Here's how the part is built. I have some questions about the finished solid (model axes, mm). Give positions to 0.01 mm unless a question says otherwise; leave off trailing zeros. Write each loop counter-clockwise with the first axis right and the second up, starting at its lowest first coordinate (ties: lowest second). Pieces come first, ordered by that corner, then holes. Notation, with made-up numbers: (-27.5, 70.5) -> (6.5, 70.5) arc R17 cw to (6.5, 101.5) -> close; hole circle Ø3 at (-23.5, 66.25). An arc over 180 degrees is marked (long way). Use one line per item in the form item = value.
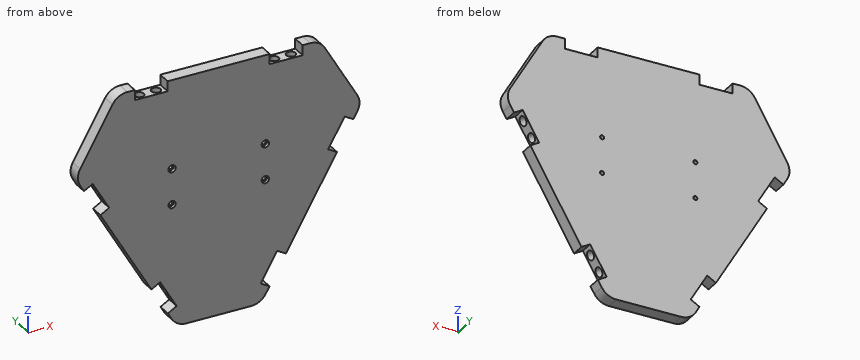
```python
from build123d import *

# Parameters (mm, degrees)
BOSS_EXTRUDE1_DEPTH            = 4
CHAMFER1_SIZE                  = 50
SKETCH4_W                      = 19.5
SKETCH4_H                      = 8
SKETCH4_R                      = 2
CUT_EXTRUDE1_DEPTH             = 6
SKETCH4_2_R                    = 2
CUT_EXTRUDE2_DEPTH             = 16
SKETCH9_R                      = 2.75
CUT_EXTRUDE3_DEPTH             = 7
CRVPATTERN1_START              = -63.508529611
CRVPATTERN1_OUTLINE_W          = 19.5
CRVPATTERN1_OUTLINE_H          = 8
CRVPATTERN1_DEPTH              = 6
CRVPATTERN1_START_2            = -57.508529611
CRVPATTERN1_2_OUTLINE_R        = 2.75
CRVPATTERN1_2_DEPTH            = 7
CRVPATTERN1_START_3            = -50.508529611
CRVPATTERN1_3_OUTLINE_R        = 2
CRVPATTERN1_3_DEPTH            = 3
CRVPATTERN1_START_4            = 57.508529611
CRVPATTERN1_4_OUTLINE_W        = 19.5
CRVPATTERN1_4_OUTLINE_H        = 8
CRVPATTERN1_4_DEPTH            = 6
CRVPATTERN1_START_5            = 50.508529611
CRVPATTERN1_5_OUTLINE_R        = 2.75
CRVPATTERN1_5_DEPTH            = 7
CRVPATTERN1_START_6            = 47.508529611
CRVPATTERN1_6_OUTLINE_R        = 2
CRVPATTERN1_6_DEPTH            = 3
FILLET1_R                      = 10
CBORE_FOR_M2_SHCS1_D           = 2.4
CBORE_FOR_M2_SHCS1_CBORE_D     = 4.4
CBORE_FOR_M2_SHCS1_CBORE_DEPTH = 2


# Read off the part's stored shape, not the designer's step: CrvPattern1
with BuildPart() as part:
    # Sketch1 → Boss-Extrude1 (new, symmetric)
    with BuildSketch(Plane(origin=(0, 0, 0), x_dir=(1, 0, 0), z_dir=(0, 1, 0))):
        Polygon((110, -63.508529611), (0, 127.017059222), (-110, -63.508529611), align=None)
    extrude(amount=BOSS_EXTRUDE1_DEPTH, both=True)

    # Chamfer1
    chamfer1_edges = [part.edges().sort_by_distance(p)[0] for p in [
        (-110, 0, 63.508529611),
        (0, 0, -127.017059222),
        (110, 0, 63.508529611),
    ]]
    chamfer(chamfer1_edges, length=CHAMFER1_SIZE)

    # Sketch4 → Cut-Extrude1 (cut)
    with BuildSketch(Plane(origin=(4.375288244, 0, 63.508529611), x_dir=(-1, 0, 0), z_dir=(0, 0, -1))):
        with Locations((44.375288244, 0)):
            Rectangle(SKETCH4_W, SKETCH4_H)
        with Locations((39.375288244, 0)):
            Circle(SKETCH4_R, mode=Mode.SUBTRACT)
        with Locations((49.375288244, 0)):
            Circle(SKETCH4_R, mode=Mode.SUBTRACT)
    cut_extrude1 = extrude(amount=CUT_EXTRUDE1_DEPTH, mode=Mode.SUBTRACT)

    # Sketch4<2> → Cut-Extrude2 (cut)
    with BuildSketch(Plane(origin=(4.375288244, 0, 63.508529611), x_dir=(-1, 0, 0), z_dir=(0, 0, -1))):
        with Locations((49.375288244, 0)):
            Circle(SKETCH4_2_R)
        with Locations((39.375288244, 0)):
            Circle(SKETCH4_2_R)
    cut_extrude2 = extrude(amount=CUT_EXTRUDE2_DEPTH, mode=Mode.SUBTRACT)

    # Sketch9 → Cut-Extrude3 (cut)
    with BuildSketch(Plane.XY.offset(57.508529611)):
        with Locations((-45, 0)):
            Circle(SKETCH9_R)
        with Locations((-35, 0)):
            Circle(SKETCH9_R)
    cut_extrude3 = extrude(amount=-CUT_EXTRUDE3_DEPTH, mode=Mode.SUBTRACT)

    # Mirror1: Cut-Extrude1, Cut-Extrude2, Cut-Extrude3 across plane
    add(cut_extrude1.mirror(Plane(origin=(0, 0, 0), x_dir=(0, 0, 1), z_dir=(1, 0, 0))), mode=Mode.SUBTRACT)
    add(cut_extrude2.mirror(Plane(origin=(0, 0, 0), x_dir=(0, 0, 1), z_dir=(1, 0, 0))), mode=Mode.SUBTRACT)
    add(cut_extrude3.mirror(Plane(origin=(0, 0, 0), x_dir=(0, 0, 1), z_dir=(1, 0, 0))), mode=Mode.SUBTRACT)

    # CrvPattern1 outline → CrvPattern1 (cut)
    with BuildSketch(Plane(origin=(0, 0, 0), x_dir=(0.499999999999987, 0, -0.8660254037844463), z_dir=(0.8660254037844461, 0, 0.49999999999998707)).offset(CRVPATTERN1_START)):
        with Locations((-40, 0)):
            Rectangle(CRVPATTERN1_OUTLINE_W, CRVPATTERN1_OUTLINE_H)
        with Locations((40, 0)):
            Rectangle(CRVPATTERN1_OUTLINE_W, CRVPATTERN1_OUTLINE_H)
    extrude(amount=CRVPATTERN1_DEPTH, mode=Mode.SUBTRACT)

    # CrvPattern1 2 outline → CrvPattern1 2 (cut)
    with BuildSketch(Plane(origin=(0, 0, 0), x_dir=(0.499999999999987, 0, -0.8660254037844463), z_dir=(0.8660254037844461, 0, 0.49999999999998707)).offset(CRVPATTERN1_START_2)):
        with Locations((-45, 0)):
            Circle(CRVPATTERN1_2_OUTLINE_R)
        with Locations((-35, 0)):
            Circle(CRVPATTERN1_2_OUTLINE_R)
        with Locations((35, 0)):
            Circle(CRVPATTERN1_2_OUTLINE_R)
        with Locations((45, 0)):
            Circle(CRVPATTERN1_2_OUTLINE_R)
    extrude(amount=CRVPATTERN1_2_DEPTH, mode=Mode.SUBTRACT)

    # CrvPattern1 3 outline → CrvPattern1 3 (cut)
    with BuildSketch(Plane(origin=(0, 0, 0), x_dir=(0.499999999999987, 0, -0.8660254037844463), z_dir=(0.8660254037844461, 0, 0.49999999999998707)).offset(CRVPATTERN1_START_3)):
        with Locations((-45, 0)):
            Circle(CRVPATTERN1_3_OUTLINE_R)
        with Locations((-35, 0)):
            Circle(CRVPATTERN1_3_OUTLINE_R)
        with Locations((35, 0)):
            Circle(CRVPATTERN1_3_OUTLINE_R)
        with Locations((45, 0)):
            Circle(CRVPATTERN1_3_OUTLINE_R)
    extrude(amount=CRVPATTERN1_3_DEPTH, mode=Mode.SUBTRACT)

    # CrvPattern1 4 outline → CrvPattern1 4 (cut)
    with BuildSketch(Plane(origin=(0, 0, 0), x_dir=(0.500000000000001, 0, 0.866025403784438), z_dir=(0.866025403784438, 0, -0.500000000000001)).offset(CRVPATTERN1_START_4)):
        with Locations((-40, 0)):
            Rectangle(CRVPATTERN1_4_OUTLINE_W, CRVPATTERN1_4_OUTLINE_H)
        with Locations((40, 0)):
            Rectangle(CRVPATTERN1_4_OUTLINE_W, CRVPATTERN1_4_OUTLINE_H)
    extrude(amount=CRVPATTERN1_4_DEPTH, mode=Mode.SUBTRACT)

    # CrvPattern1 5 outline → CrvPattern1 5 (cut)
    with BuildSketch(Plane(origin=(0, 0, 0), x_dir=(0.500000000000001, 0, 0.866025403784438), z_dir=(0.866025403784438, 0, -0.500000000000001)).offset(CRVPATTERN1_START_5)):
        with Locations((-45, 0)):
            Circle(CRVPATTERN1_5_OUTLINE_R)
        with Locations((-35, 0)):
            Circle(CRVPATTERN1_5_OUTLINE_R)
        with Locations((35, 0)):
            Circle(CRVPATTERN1_5_OUTLINE_R)
        with Locations((45, 0)):
            Circle(CRVPATTERN1_5_OUTLINE_R)
    extrude(amount=CRVPATTERN1_5_DEPTH, mode=Mode.SUBTRACT)

    # CrvPattern1 6 outline → CrvPattern1 6 (cut)
    with BuildSketch(Plane(origin=(0, 0, 0), x_dir=(0.500000000000001, 0, 0.866025403784438), z_dir=(0.866025403784438, 0, -0.500000000000001)).offset(CRVPATTERN1_START_6)):
        with Locations((-45, 0)):
            Circle(CRVPATTERN1_6_OUTLINE_R)
        with Locations((-35, 0)):
            Circle(CRVPATTERN1_6_OUTLINE_R)
        with Locations((35, 0)):
            Circle(CRVPATTERN1_6_OUTLINE_R)
        with Locations((45, 0)):
            Circle(CRVPATTERN1_6_OUTLINE_R)
    extrude(amount=CRVPATTERN1_6_DEPTH, mode=Mode.SUBTRACT)

    # Fillet1
    fillet1_edges = [part.edges().sort_by_distance(p)[0] for p in [
        (60, 0, 63.508529611),
        (-60, 0, 63.508529611),
        (-25, 0, -83.715789032),
        (-85, 0, 20.207259422),
        (25, 0, -83.715789032),
        (85, 0, 20.207259422),
    ]]
    fillet(fillet1_edges, radius=FILLET1_R)

    # CBORE for M2 SHCS1 (through all)
    with Locations(Plane(origin=(0, -4, 0), x_dir=(-1, 0, 0), z_dir=(0, -1, 0))):
        with Locations((-27.65, -10.65), (27.65, 10.65), (27.65, -10.65), (-27.65, 10.65)):
            CounterBoreHole(CBORE_FOR_M2_SHCS1_D / 2, CBORE_FOR_M2_SHCS1_CBORE_D / 2, CBORE_FOR_M2_SHCS1_CBORE_DEPTH)


solid = part.part
```
Q1. I want a section at B-B, the plane x = -45. Write out the boundary of the cut face in (y, z).
Result set:
outline = (-4, -49.07) -> (4, -49.07) -> (4, 57.51) -> (2.75, 57.51) -> (2.75, 50.51) -> (2, 50.51) -> (2, 47.51) -> (-2, 47.51) -> (-2, 50.51) -> (-2.75, 50.51) -> (-2.75, 57.51) -> (-4, 57.51) -> close
Q2. If I drill on line 1 along X through (y, z) = (-3.35, -10.65); line 2 along X through (y, z) = (-0.35, -10.65); line 3 along Z through (x, y) = (-69.5, 2), over which ranges is the centre line in solid material (lowest first)? Write a range as from..to.
Result set:
line_1 = -67.18..-29.85, -25.45..25.45, 29.85..67.18
line_2 = -67.18..-28.85, -26.45..26.45, 28.85..67.18
line_3 = -6.64..-5.2, 5.36..9.66, 14.02..47.05
Q3. I want a section at A-A, the plane z = 55. Write out the boundary of the cut face in (x, y), and give its area (3 significant figures).
Result set:
outline = (-64.91, -4) -> (64.91, -4) -> (64.91, 4) -> (-64.91, 4) -> close; hole circle Ø5.5 at (-45, 0); hole circle Ø5.5 at (-35, 0); hole circle Ø5.5 at (35, 0); hole circle Ø5.5 at (45, 0)
area = 944 mm2
Q4. I want a section at C-C, the plane z = -50. Write out the boundary of the cut face in (x, y), and give its area (3 significant figures).
Result set:
outline = (-44.47, -4) -> (44.47, -4) -> (44.47, 4) -> (-44.47, 4) -> close
area = 711 mm2
Q5. Will these pins go through, and if not, where does the flat tip stop? pin 1 Ø4.5 at (x, y) = (-35, 0) entering from -Z; pin 2 Ø3.5 at (x, z) = (27.65, 10.65) entering from -Y; pin 3 Ø4 at (x, z) = (27.65, -10.65) entering from +Y; pin 4 Ø1 at (x, y) = (-46.5, -3) entering from -Z.
Result set:
pin_1 = -57.13
pin_2 = -2
pin_3 = 4
pin_4 = -47.34
